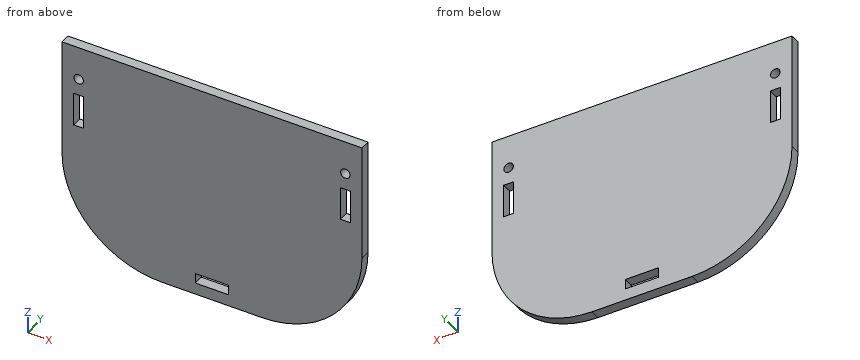
```python
from build123d import *

# Parameters (mm, degrees)
SKETCH1_W           = 90
SKETCH1_H           = 65
SKETCH1_R           = 1.425
SKETCH1_W_2         = 10
SKETCH1_H_2         = 3
SKETCH1_W_3         = 3
SKETCH1_H_3         = 10
BOSS_EXTRUDE1_DEPTH = 3
FILLET1_R           = 30


with BuildPart() as part:
    # Sketch1 → Boss-Extrude1 (new body)
    with BuildSketch(Plane(origin=(0, 0, 0), x_dir=(1, 0, 0), z_dir=(0, 1, 0))):
        with Locations((0, 27.5)):
            Rectangle(SKETCH1_W, SKETCH1_H)
        with Locations(Location((-40, 5, 0), (0, 0, 270))):
            Circle(SKETCH1_R, mode=Mode.SUBTRACT)
        with Locations(Location((40, 5, 0), (0, 0, 270))):
            Circle(SKETCH1_R, mode=Mode.SUBTRACT)
        with Locations((0, 55)):
            Rectangle(SKETCH1_W_2, SKETCH1_H_2, mode=Mode.SUBTRACT)
        with Locations((-40, 15)):
            Rectangle(SKETCH1_W_3, SKETCH1_H_3, mode=Mode.SUBTRACT)
        with Locations((40, 15)):
            Rectangle(SKETCH1_W_3, SKETCH1_H_3, mode=Mode.SUBTRACT)
    extrude(amount=BOSS_EXTRUDE1_DEPTH)

    # Fillet1
    fillet1_edges = [part.edges().sort_by_distance(p)[0] for p in [
        (-45, 1.5, -60),
        (45, 1.5, -60),
    ]]
    fillet(fillet1_edges, radius=FILLET1_R)


solid = part.part
```
Could you check a few things on this model? Use its own coordinates, in mm. Round coordinates to 2 decimals unless told otherwise and drop trailing zeros. Write each loop counter-clockwise with the first axis right and the second up, starting at its lowest first coordinate (ties: lowest second). Pieces come first, ordered by that corner, then holes. Notation, with made-up numbers: M -11,-37 L 45,-37 A36 ccw 45,0 Z; hole C -1,-36 d8. An arc over 180 degrees is marked long. Write each question's results on one line, items separated by ' | '. Start each with the question number.
1. I need wall thicknesses on L1, parallel to X at y = 1.7, z = -5 (3 decimals); L2, parallel to X at y = 2.6, z = -4.5; L3, parallel to X at y = 2.6, z = -56. Which ranges of each line are inside material? Lowest first, please. Write a range as from..to.
2. I'm going to push a flat-ended pin straight in: pin 1 Ø4.5 at (x, z) = (-40, -5) entering from +Y. Where does the tip first touch, or does it pass through?
3. Imagine slicing it at A-A on z = -5. List the corners of the cut face in (x, y) for me (3 decimals).
4. Imagine slicing it at B-B on x = -40. List the corners of the cut face in (y, z) for me (3 decimals).
5. Imagine slicing it at D-D on z = -48. List the corners of the cut face in (x, y) for me.
6. Imagine slicing it at C-C on y = 1.05. List the corners of the cut face in (x, z) for me (3 decimals).
Result sheet:
1) L1: x = -45..-41.425, -38.575..38.575, 41.425..45 | L2: x = -45..-41.33, -38.67..38.67, 41.33..45 | L3: x = -29.97..-5, 5..29.97
2) pin 1: stops at y = 3
3) outline: M -45,0 L -41.425,0 L -41.425,3 L -45,3 Z; M -38.575,0 L 38.575,0 L 38.575,3 L -38.575,3 Z; M 41.425,0 L 45,0 L 45,3 L 41.425,3 Z
4) outline: M 0,-46.583 L 3,-46.583 L 3,-20 L 0,-20 Z; M 0,-10 L 3,-10 L 3,-6.425 L 0,-6.425 Z; M 0,-3.575 L 3,-3.575 L 3,5 L 0,5 Z
5) outline: M -39,0 L 39,0 L 39,3 L -39,3 Z
6) outline: M -45,-30 A30 ccw -15,-60 L 15,-60 A30 ccw 45,-30 L 45,5 L -45,5 Z; hole M -41.5,-20 L -38.5,-20 L -38.5,-10 L -41.5,-10 Z; hole C -40,-5 d2.85; hole M -5,-56.5 L 5,-56.5 L 5,-53.5 L -5,-53.5 Z; hole M 38.5,-20 L 41.5,-20 L 41.5,-10 L 38.5,-10 Z; hole C 40,-5 d2.85
